Autodesk Inventor part; units mm, degrees
ref_plane "Work Plane2" through (-60.0293, 37.0443, -153.2141) normal (-1, 0, 0) x (0, 0, 1)
ref_plane "YZ Plane" through (0, 0, 0) normal (1, 0, 0) x (0, 1, 0)
ref_plane "XZ Plane" through (0, 0, 0) normal (0, 1, 0) x (-1, 0, 0)
ref_plane "Work Plane1" through (-60.0293, 37.0443, 146.7859) normal (0, 0, 1) x (1, 0, 0)
sketch "Sketch1" plane through (-60.0293, 37.0443, 146.7859) normal (0, 0, 1) x (1, 0, 0)
  line L0 (55.8868, 5) -> (53, 0)
  line L1 (53, 0) -> (60, 0)
  line L2 (60, 0) -> (60, 10)
  line L3 (20, 10) -> (60, 10)
  line L4 (20, 10) -> (20, 40)
  line L5 (0, 40) -> (20, 40)
  line L6 (0, 0) -> (0, 40)
  line L7 (0, 0) -> (7, 0)
  line L8 (7, 0) -> (4.1132, 5)
  line L9 (4.1132, 5) -> (19.8868, 5)
  line L10 (19.8868, 5) -> (17, 0)
  line L11 (17, 0) -> (43, 0)
  line L12 (43, 0) -> (40.1132, 5)
  line L13 (40.1132, 5) -> (55.8868, 5)
  circle A0 centre (10, 32) radius 6
  line L14 (0, 0) -> (60, 0)
  line L15 (60, 0) -> (60, -100)
  line L16 (60, -100) -> (0, -100)
  line L17 (0, -100) -> (0, 0)
  point P0 (60.0293, -37.0443)
  dimension "d0" = 60
  dimension "d1" = 100
extrude "Extrusion1" add sketch "Sketch1" along normal blind 10 contours L0 L14 L12 L13 | L1 L15 L16 L17 L7 L14 L11 | L14 L8 L9 L10
sketch "Sketch2" plane through (-43.0293, 37.0443, 146.7859) normal (0, 1, 0) x (1, 0, 0)
  line L0 (17, -10) -> (9, -10)
  line L1 (9, -10) -> (9, 0)
  line L2 (9, 0) -> (17, 0)
  line L3 (17, 0) -> (17, -10)
  line L4 (17, -10) -> (9, 0) construction
  line L5 (9, -10) -> (17, 0) construction
  line L6 (55.0352, 0) -> (-29.0059, 0)
  line L7 (43, 0) -> (43, -10)
  point P0 (43.0293, 146.7859)
  point P1 (13, -5)
  dimension "d4" = 8
  dimension "d5" = 10
  dimension "d6" = 0
  dimension "d9" = 30
extrude "Extrusion2" add sketch "Sketch2" along normal up to surface (40 mm away)
sketch "Sketch3" plane through (-34.0293, 37.0443, 146.7859) normal (-1, 0, 0) x (0, 0, 1)
  line L0 (10, 40) -> (0, 40)
  line L1 (0, 0) -> (0, 40)
  line L2 (10, 0) -> (0, 0)
  line L3 (10, 0) -> (10, 40)
  line L4 (0, 0) -> (0, 40)
  line L5 (0, 20) -> (10, 20)
  point P0 (-146.7859, -37.0443)
  point P1 (0, 20)
  dimension "d10" = 20
ref_plane "Work Plane2" through (-60.0293, 37.0443, -153.2141) normal (-1, 0, 0) x (0, 0, 1)
extrude "Extrusion3" add sketch "Sketch3" along normal up to surface (26 mm away) contours L3 L5 L1 L0
sketch "Sketch4" plane through (-60.0293, 37.0443, 156.7859) normal (0, 0, 1) x (1, 0, 0)
  circle A0 centre (10, 32) radius 6
  point P0 (60.0293, -37.0443)
extrude "Extrusion4" cut sketch "Sketch4" against normal through all
thread "Thread1"
properties part number "jaws"
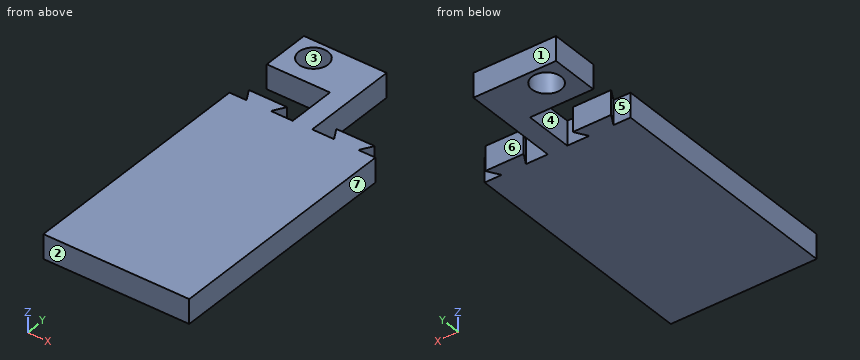
Input: part model. Units: mm. Frame: model coordinates. Face numbers are marked on the shaded views. A direction names the side the tool comes from. Give positions to 0.01 mm unless a question says otherwise; leave off trailing zeros. Order: outer loops, then holes, each group sorted by start corner. A loop starts at its lowest first (then second) coordinate and runs counter-clockwise, first axis right, second up. Notation, with made-up numbers: M 50.5,6.5 L 61.5,6.5 A19 cw 61.5,31.5 Z; hole C 81,48 d6. An arc over 180 degrees is marked long. One line per question, with ' | ' between items.
1) Section C-C on z = 148.25. Output: boundary loops of the cut face in (x, y).
Filled in:
outline: M -60.03,-62.96 L -0.03,-62.96 L -0.03,37.04 L -7.03,37.04 L -4.14,42.04 L -19.92,42.04 L -17.03,37.04 L -26.03,37.04 L -26.03,77.04 L -60.03,77.04 L -60.03,57.04 L -34.03,57.04 L -34.03,37.04 L -43.03,37.04 L -40.14,42.04 L -55.92,42.04 L -53.03,37.04 L -60.03,37.04 Z; hole C -50.03,69.04 d12
2) Section B-B on y = 65. Output: boundary loops of the cut face in (x, z), and give its area (3 significant figures).
Filled in:
outline: M -60.03,146.79 L -54.46,146.79 L -54.46,156.79 L -60.03,156.79 Z; M -45.6,146.79 L -26.03,146.79 L -26.03,156.79 L -45.6,156.79 Z | area: 251 mm2
3) Access query for the marked faces 4, 5, 6 and 7. Directions: +Z, -Z, +X, -X, +Y, -Y. A direction counts if a zero-diameter tool reaches every point of the face in a straight line with its end or side. Return the directions, or none.
Filled in:
face 4: +Z, -Z | face 5: +Z, -Z, -X | face 6: +Z, -Z, +X, +Y | face 7: +Z, -Z, +X, +Y, -Y
4) Section D-D on x = -12. Output: boundary loops of the cut face in (y, z).
Filled in:
outline: M -62.96,146.79 L 42.04,146.79 L 42.04,156.79 L -62.96,156.79 Z
5) Draft query along Y for the marked faces 1, 2 and 3. Return one class per face: pulls with the +Y half, pulls with the -Y half, needs draft (parallel to the pull), parting line crosses it, or undercut.
Filled in:
face 1: pulls with the +Y half | face 2: pulls with the -Y half | face 3: undercut
6) Contact query for flat-ended pins moving along their axis: P1, Ø5, axis at x = -15.5, z = 151.5, coming from the +Y side; P2, Ø15.5, axis at x = -50.03, y = 69.04, coming from the -Z side; P3, Ø5, axis at y = 51, z = 153.5, coming from the +X side. Output: stop coordinate, or through.
Filled in:
P1: stops at y = 42.04 | P2: stops at z = 146.79 | P3: stops at x = -26.03
7) Section A-A on x = -18.5. Output: boundary loops of the cut face in (y, z), and give its area (3 significant figures).
Filled in:
outline: M -62.96,146.79 L 37.04,146.79 L 37.04,156.79 L -62.96,156.79 Z; M 39.59,146.79 L 42.04,146.79 L 42.04,156.79 L 39.59,156.79 Z | area: 1,020 mm2
8) Ray query, L1, parallel to Y at x = -49.5, z = 153.5; L2, parallel to Y at x = -39, z = 154; L3, parallel to Y at x = -47.5, z = 149.75. Return the intervals inside material, ascending.
Filled in:
L1: y = -62.96 to 42.04, 57.04 to 63.07, 75.02 to 77.04 | L2: y = -62.96 to 37.04, 57.04 to 77.04 | L3: y = -62.96 to 42.04, 57.04 to 63.6, 74.49 to 77.04
